from build123d import *

# Parameters (mm, degrees)
SKETCH1_W           = 97.028
SKETCH1_H           = 21.59
SKETCH1_R           = 1.778
BOSS_EXTRUDE1_DEPTH = 0.635
BOSS_EXTRUDE2_DEPTH = 34.29
BOSS_EXTRUDE3_DEPTH = 7.62


with BuildPart() as part:
    # Sketch1 → Boss-Extrude1 (new, symmetric)
    with BuildSketch(Plane(origin=(0, 0, 0), x_dir=(1, 0, 0), z_dir=(0, 1, 0))):
        Rectangle(SKETCH1_W, SKETCH1_H)
        with Locations(Location((-44.831, 0, 0), (0, 0, 270))):
            Circle(SKETCH1_R, mode=Mode.SUBTRACT)
        with Locations(Location((44.831, 0, 0), (0, 0, 90))):
            Circle(SKETCH1_R, mode=Mode.SUBTRACT)
    extrude(amount=BOSS_EXTRUDE1_DEPTH, both=True)

    # Sketch2 → Boss-Extrude2 (add, symmetric)
    with BuildSketch(Plane(origin=(0, 0, 0), x_dir=(0, 0, -1), z_dir=(1, 0, 0))):
        Polygon((-10.541, 0.635), (-10.541, 10.16), (-9.652, 10.16), (-8.465143093, 16.891), (-2.314009226, 16.891), (0, 8.255), (2.314009226, 16.891), (8.465143093, 16.891), (9.652, 10.16), (10.541, 10.16), (10.541, 0.635), align=None)
    extrude(amount=BOSS_EXTRUDE2_DEPTH, both=True)

    # Sketch3 → Boss-Extrude3 (add, symmetric)
    with BuildSketch(Plane.XY):
        Polygon((-34.798, 0.635), (-34.798, 8.255), (-35.553552098, 16.891), (-40.393571647, 16.891), (-41.580428554, 10.16), (-42.596428554, 10.16), (-42.596428554, 0.635), align=None)
    boss_extrude3 = extrude(amount=BOSS_EXTRUDE3_DEPTH, both=True)

    # Mirror1: Boss-Extrude3 across plane
    add(boss_extrude3.mirror(Plane(origin=(0, 0, 0), x_dir=(0, 0, 1), z_dir=(1, 0, 0))))


solid = part.part
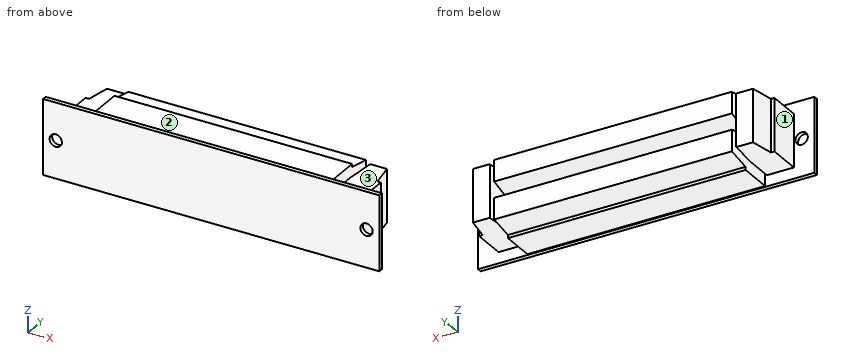
Geometry check sheet. Reference: the model listing, model coordinates, mm. Face numbers are marked on the shaded views. A direction names the side the tool comes from. Give positions to 0.01 mm unless a question says otherwise; leave off trailing zeros. Order: outer loops, then holes, each group sorted by start corner. A loop starts at its lowest first (then second) coordinate and runs counter-clockwise, first axis right, second up.
1. Depth check by flat-ended pin: pin 1 (2 mm diameter, centred on y = 10.5, z = -6, fed in from +X); pin 2 (2.5 mm diameter, centred on y = 5.5, z = 2, fed in from -X); pin 3 (8.5 mm diameter, centred on x = -40.5, y = 10, fed in from +Z). Enter the tip coordinate at first touch or a pass-through.
Completed:
pin 1: stops at x = 42.6
pin 2: stops at x = -42.6
pin 3: stops at z = 7.62
2. Sectioned sample at A-A (y = 5.25). Record the boundary of the cut face in (x, z), then the cut area to 3 significant figures.
Completed:
outline: (-42.6, -7.62) - (-34.8, -7.62) - (-34.8, 7.62) - (-42.6, 7.62) - close; (-34.29, -10.54) - (34.29, -10.54) - (34.29, 10.54) - (-34.29, 10.54) - close; (34.8, -7.62) - (42.6, -7.62) - (42.6, 7.62) - (34.8, 7.62) - close
area: 1,680 mm2
3. Sectioned sample at D-D (z = -3.5). Record the boundary of the cut face in (x, y) (3 decimals), then the cut area to 3 significant figures.
Completed:
outline: (-48.514, -0.635) - (48.514, -0.635) - (48.514, 0.635) - (42.596, 0.635) - (42.596, 10.16) - (41.58, 10.16) - (40.394, 16.891) - (35.554, 16.891) - (34.798, 8.255) - (34.798, 0.635) - (34.29, 0.635) - (34.29, 16.891) - (-34.29, 16.891) - (-34.29, 0.635) - (-34.798, 0.635) - (-34.798, 8.255) - (-35.554, 16.891) - (-40.394, 16.891) - (-41.58, 10.16) - (-42.596, 10.16) - (-42.596, 0.635) - (-48.514, 0.635) - close
area: 1,460 mm2
4. Scan lines: line 1 (X direction, y = -0.3, z = 0); line 2 (X direction, y = 1.75, z = 6.5); line 3 (Z direction, x = -21, y = 0.75). Record each from-to range of solid material in increasing order.
Completed:
line 1: x = -48.51 to -46.61, -43.05 to 43.05, 46.61 to 48.51
line 2: x = -42.6 to -34.8, -34.29 to 34.29, 34.8 to 42.6
line 3: z = -10.54 to 10.54
5. Access from +Z, -Z, +X, -X, +Y, -Y to the whole of each face (thin tool, end or side, straight path). Record for the marked faces 1, 2 and 3.
Completed:
face 1: +Z, -Z, -X, +Y
face 2: +Z, +X, -X, +Y
face 3: +Z, +X, +Y
6. Sectioned sample at B-B (y = 11.75). Record the boundary of the cut face in (x, z).
Completed:
outline: (-41.3, -7.62) - (-35.1, -7.62) - (-35.1, 7.62) - (-41.3, 7.62) - close; (-34.29, -9.37) - (34.29, -9.37) - (34.29, -0.94) - (-34.29, -0.94) - close; (-34.29, 0.94) - (34.29, 0.94) - (34.29, 9.37) - (-34.29, 9.37) - close; (35.1, -7.62) - (41.3, -7.62) - (41.3, 7.62) - (35.1, 7.62) - close
7. Sectioned sample at C-C (x = -15.5). Record the boundary of the cut face in (y, z) (3 decimals).
Completed:
outline: (-0.635, -10.795) - (0.635, -10.795) - (0.635, -10.541) - (10.16, -10.541) - (10.16, -9.652) - (16.891, -8.465) - (16.891, -2.314) - (8.255, 0) - (16.891, 2.314) - (16.891, 8.465) - (10.16, 9.652) - (10.16, 10.541) - (0.635, 10.541) - (0.635, 10.795) - (-0.635, 10.795) - close
